Autodesk Inventor part; units mm, degrees
ref_plane "PulleyMidPlane1" through (-30.1251, 9, -4) normal (1, 0, 0) x (0, 0, -1)
ref_plane "PulleyMidPlane2" through (-23.3752, 9, -4) normal (1, 0, 0) x (0, 0, -1)
ref_plane "YZ Plane" through (0, 0, 0) normal (1, 0, 0) x (0, 1, 0)
sketch "Sketch1" plane through (0, 0, 0) normal (0, 1, 0) x (-1, 0, 0)
  line L0 (0, 0) -> (35.5, 0)
  line L1 (35.5, 0) -> (35.5, -90)
  line L2 (35.5, -90) -> (0, -90)
  line L3 (0, -90) -> (0, 0)
  dimension "d0" = 35.5
  dimension "d1" = 90
extrude "BlockShape" add sketch "Sketch1" along normal blind 9
sketch "Sketch3" plane through (0, 0, 0) normal (0, -1, 0) x (1, 0, 0)
  circle A0 centre (-10, -25) radius 3.25 construction
  line L0 (0, 0) -> (-35.5, 0)
  line L1 (-35.5, 0) -> (-35.5, -90)
  line L2 (-11.6286, -27.8125) -> (-13.25, -24.9958)
  line L3 (-13.25, -24.9958) -> (-11.6214, -22.1833)
  line L4 (-11.6214, -22.1833) -> (-8.3714, -22.1875)
  line L5 (-8.3714, -22.1875) -> (-6.75, -25.0042)
  line L6 (-6.75, -25.0042) -> (-8.3786, -27.8167)
  line L7 (-8.3786, -27.8167) -> (-11.6286, -27.8125)
  line L8 (0, -90) -> (0, 0)
  dimension "d15" = 6.5
  dimension "d16" = 25
  dimension "d26" = 10
extrude "SlideMountingNutWell1" cut sketch "Sketch3" against normal blind 5
sketch "Sketch5" plane through (0, 9, 0) normal (0, 1, 0) x (1, 0, 0)
  line L0 (0, 0) -> (0, 90)
  line L1 (-35.5, 0) -> (0, 0)
  circle A0 centre (-10, 25) radius 1.7
  circle A1 centre (-10, 15) radius 1.7
  dimension "d36" = 3.4
  dimension "d37" = 25
  dimension "d137" = 3.4
  dimension "d138" = 15
extrude "SlideMountingHoles" cut sketch "Sketch5" against normal through all
sketch "Sketch6" plane through (0, 9, 0) normal (0, 1, 0) x (1, 0, 0)
  line L0 (-32.5, 4) -> (-27.7502, 4)
  line L1 (-27.7502, 4) -> (-27.7502, 29.4)
  line L2 (-27.7502, 29.4) -> (-32.5, 29.4)
  line L3 (-32.5, 29.4) -> (-32.5, 4)
  line L4 (-35.5, 0) -> (0, 0)
  line L5 (-35.5, 90) -> (-35.5, 0)
  line L6 (-25.7502, 4) -> (-21.0002, 4)
  line L7 (-21.0002, 4) -> (-21.0002, 16.7)
  line L8 (-21.0002, 16.7) -> (-25.7502, 16.7)
  line L9 (-25.7502, 16.7) -> (-25.7502, 4)
  line L10 (0, 0) -> (0, 90) construction
  line L11 (-35.5, 90) -> (0, 90)
  line L12 (0, 0) -> (-20, 0) construction
  line L13 (-20, 0) -> (-20, 90) construction
  line L14 (-20, 90) -> (0, 90) construction
  line L15 (0, 90) -> (0, 0)
  circle A0 centre (-23.3752, 41.7) radius 1.7
  circle A1 centre (-30.125, 41.7) radius 1.7
  circle A2 centre (-30.125, 49.7) radius 1.7
  circle A3 centre (-23.3752, 49.7) radius 1.7
  dimension "d43" = 4.7498
  dimension "d44" = 25.4
  dimension "d45" = 4
  dimension "d46" = 3
  dimension "d47" = 4.75
  dimension "d48" = 2
  dimension "d49" = 20
  dimension "d50" = 3.4
  dimension "d90" = 3.4
  dimension "d91" = 5.375
  dimension "d92" = 3.4
  dimension "d93" = 8
  dimension "d94" = 3.4
  dimension "d99" = 40.3
extrude "Shape" cut sketch "Sketch6" against normal through all contours L3 L2 L1 L0 | L9 L8 L7 L6 | A0 | A1 | A2 | A3
sketch "Sketch7" plane through (0, 0, 0) normal (0, -1, 0) x (1, 0, 0)
  circle A0 centre (-23.3752, -41.7) radius 1.7
  circle A1 centre (-23.3752, -41.7) radius 3.25 construction
  line L0 (-23.3752, -38.45) -> (-20.5606, -40.075)
  line L1 (-20.5606, -40.075) -> (-20.5606, -43.325)
  line L2 (-20.5606, -43.325) -> (-23.3752, -44.95)
  line L3 (-23.3752, -44.95) -> (-26.1898, -43.325)
  line L4 (-26.1898, -43.325) -> (-26.1898, -40.075)
  line L5 (-26.1898, -40.075) -> (-23.3752, -38.45)
  line L6 (0, 0) -> (-35.5, 0)
  circle A2 centre (-30.125, -41.7) radius 3.25 construction
  line L7 (-35.5, 0) -> (-35.5, -90)
  line L8 (-30.1645, -44.9498) -> (-32.9591, -43.2907)
  line L9 (-32.9591, -43.2907) -> (-32.9196, -40.0409)
  line L10 (-32.9196, -40.0409) -> (-30.0855, -38.4502)
  line L11 (-30.0855, -38.4502) -> (-27.2909, -40.1093)
  line L12 (-27.2909, -40.1093) -> (-27.3304, -43.3591)
  line L13 (-27.3304, -43.3591) -> (-30.1645, -44.9498)
  dimension "d88" = 6.5
  dimension "d54" = 6.5
  dimension "d87" = 41.7
  dimension "d89" = 5.375
extrude "TensionNutWells1" cut sketch "Sketch7" against normal blind 5
sketch "Sketch8" plane through (-35.5, 0, -90) normal (-1, 0, 0) x (0, 0, 1)
  circle A0 centre (79.65, 4.5) radius 1.4605
  line L0 (0, 9) -> (90, 9)
  line L1 (90, 0) -> (90, 9)
  circle A1 centre (66.95, 4.5) radius 1.4605
  dimension "d57" = 2.921
  dimension "d58" = 4.5
  dimension "d59" = 10.35
  dimension "d103" = 2.921
  dimension "d104" = 4.5
  dimension "d105" = 12.7
hole "PulleyMountingHoles" at (-35.5, 4.5, -10.35) at (-35.5, 4.5, -23.05) direction (1, 0, 0) diameter 2.921 depth 22.5 counterbore diameter 3.4 counterbore depth 1.5
sketch "Sketch9" plane through (-21.0002, 9, -16.7) normal (-1, 0, 0) x (0, 0, 1)
  circle A0 centre (6.35, -4.5) radius 1.4605
  circle A1 centre (6.35, -4.5) radius 2.54
  point P0 (16.7, -9)
  dimension "d67" = 5.08
extrude "PulleyStandoff1" add sketch "Sketch9" along normal blind 0.2032
sketch "Sketch10" plane through (-27.7502, 9, -29.4) normal (-1, 0, 0) x (0, 0, 1)
  circle A0 centre (6.35, -4.5) radius 1.7
  circle A1 centre (6.35, -4.5) radius 2.54
  circle A2 centre (19.05, -4.5) radius 2.54
  circle A3 centre (19.05, -4.5) radius 2.54
  circle A4 centre (19.05, -4.5) radius 1.7
  point P0 (29.4, -9)
  dimension "d70" = 5.08
  dimension "d106" = 3.4
extrude "PulleyStandoff3" add sketch "Sketch10" along normal blind 0.2032
sketch "Sketch11" plane through (-25.7502, 9, -4) normal (1, 0, 0) x (0, 0, -1)
  circle A0 centre (6.35, -4.5) radius 1.7
  circle A1 centre (6.35, -4.5) radius 2.54
  point P0 (-4, -9)
  dimension "d73" = 5.08
extrude "PulleyStandoff2" add sketch "Sketch11" along normal blind 0.2032
sketch "Sketch12" plane through (-32.5, 9, -4) normal (1, 0, 0) x (0, 0, -1)
  circle A0 centre (6.35, -4.5) radius 1.7
  circle A1 centre (6.35, -4.5) radius 2.54
  circle A2 centre (19.05, -4.5) radius 1.4605
  circle A3 centre (19.05, -4.5) radius 2.54
  circle A4 centre (19.05, -4.5) radius 1.7
  point P0 (-4, -9)
  dimension "d76" = 5.08
  dimension "d107" = 5.08
  dimension "d108" = 3.4
extrude "PulleyStandof4" add sketch "Sketch12" along normal blind 0.2032 contours A1 | A3
sketch "Sketch14" plane through (0, 0, -90) normal (0, 0, -1) x (-1, 0, 0)
  circle A0 centre (18, 4.5) radius 2.25
  line L0 (35.5, 0) -> (0, 0)
  line L1 (0, 0) -> (0, 9)
  dimension "d82" = 4.5
  dimension "d83" = 4.5
  dimension "d84" = 18
extrude "4mmShaft" cut sketch "Sketch14" against normal blind 41
sketch "Sketch15" plane through (0, 9, 0) normal (0, 1, 0) x (1, 0, 0)
  circle A0 centre (-30.125, 49.7) radius 1.7
  circle A1 centre (-30.125, 49.7) radius 3.25 construction
  circle A2 centre (-23.3752, 49.7) radius 1.7
  circle A3 centre (-23.3752, 49.7) radius 3.25 construction
  line L0 (-30.125, 52.95) -> (-27.3104, 51.325)
  line L1 (-27.3104, 51.325) -> (-27.3104, 48.075)
  line L2 (-27.3104, 48.075) -> (-30.125, 46.45)
  line L3 (-30.125, 46.45) -> (-32.9396, 48.075)
  line L4 (-32.9396, 48.075) -> (-32.9396, 51.325)
  line L5 (-32.9396, 51.325) -> (-30.125, 52.95)
  line L6 (-23.3752, 52.95) -> (-20.5606, 51.325)
  line L7 (-20.5606, 51.325) -> (-20.5606, 48.075)
  line L8 (-20.5606, 48.075) -> (-23.3752, 46.45)
  line L9 (-23.3752, 46.45) -> (-26.1898, 48.075)
  line L10 (-26.1898, 48.075) -> (-26.1898, 51.325)
  line L11 (-26.1898, 51.325) -> (-23.3752, 52.95)
  point P0 (0, 0)
  dimension "d95" = 6.5
  dimension "d96" = 6.5
extrude "TensionNutWells2" cut sketch "Sketch15" against normal blind 5
ref_plane "PulleyMidPlane1" through (-30.1251, 9, -4) normal (1, 0, 0) x (0, 0, -1)
ref_plane "PulleyMidPlane2" through (-23.3752, 9, -4) normal (1, 0, 0) x (0, 0, -1)
sketch "Sketch20" plane through (0, 9, 0) normal (0, 1, 0) x (1, 0, 0)
  circle A0 centre (-29.5, 86) radius 1.524
  circle A1 centre (-29.5, 57.7) radius 1.524
  line L0 (-35.5, 90) -> (-35.5, 0)
  line L1 (0, 90) -> (-35.5, 90)
  circle A2 centre (-30.125, 49.7) radius 1.7
  point P0 (0, 0)
  dimension "d129" = 3.048
  dimension "d130" = 3.048
  dimension "d131" = 6
  dimension "d132" = 4
  dimension "d133" = 6
  dimension "d134" = 8
extrude "TieWrapHoles" cut sketch "Sketch20" against normal through all contours A0 | A1
sketch "Sketch21" plane through (0, 9, 0) normal (0, 1, 0) x (1, 0, 0)
  circle A0 centre (-10, 15) radius 1.7 construction
  circle A1 centre (-10, 15) radius 3.25 construction
  line L0 (-6.75, 15) -> (-8.375, 12.1854)
  line L1 (-8.375, 12.1854) -> (-11.625, 12.1854)
  line L2 (-11.625, 12.1854) -> (-13.25, 15)
  line L3 (-13.25, 15) -> (-11.625, 17.8146)
  line L4 (-11.625, 17.8146) -> (-8.375, 17.8146)
  line L5 (-8.375, 17.8146) -> (-6.75, 15)
  point P0 (0, 0)
  dimension "d139" = 6.5
extrude "SlideMountingNutWell2" cut sketch "Sketch21" against normal blind 5
sketch "Sketch22" plane through (0, 0, 0) normal (0, -1, 0) x (1, 0, 0)
  circle A0 centre (-9.525, -35) radius 1.9304 construction
  circle A1 centre (-9.525, -54.558) radius 1.9304 construction
  circle A2 centre (-10, -25) radius 1.7 construction
  line L0 (0, -90) -> (0, 0) construction
  dimension "d142" = 3.8608
  dimension "d143" = 3.8608
  dimension "d144" = 19.558
  dimension "d145" = 9.525
  dimension "d146" = 10
hole "XRrailMountingHoles1" at (-9.525, 0, -54.558) at (-9.525, 0, -35) direction (0, 1, 0) diameter 3.8608 end through all counterbore diameter 8.89 counterbore depth 3.048
sketch "Sketch23" plane through (0, 9, 0) normal (0, 1, 0) x (1, 0, 0)
  circle A0 centre (-9.525, 44.779) radius 1.9304 construction
  circle A1 centre (-9.525, 64.337) radius 1.9304 construction
  circle A2 centre (-9.525, 35) radius 1.9304
  line L0 (0, 0) -> (0, 90)
  dimension "d154" = 3.8608
  dimension "d155" = 3.8608
  dimension "d156" = 19.558
  dimension "d157" = 9.779
  dimension "d158" = 9.525
hole "XRrailMountingHoles2" at (-9.525, 9, -44.779) at (-9.525, 9, -64.337) direction (0, -1, 0) diameter 3.8608 end through all counterbore diameter 8.89 counterbore depth 3.048
sketch "Sketch25" plane through (0, 0, 0) normal (1, 0, 0) x (0, 0, -1)
  circle A0 centre (6.65, 4.5) radius 1.45
  line L0 (90, 0) -> (0, 0) construction
  line L1 (0, 9) -> (90, 9) construction
  line L2 (13.3, 4) -> (13.3, 0) construction
  line L3 (0, 0) -> (0, 9) construction
  line L4 (66.2674, 5.952) -> (62.4066, 5.952) construction
  line L5 (59.892, 9) -> (68.782, 9) construction
  line L6 (68.782, 5.952) -> (59.892, 5.952) construction
  line L7 (90, 0) -> (90, 9) construction
  circle A1 centre (75.8547, 4.5) radius 1.45
  circle A2 centre (82.9273, 4.5) radius 1.45
  dimension "d178" = 2.9
  dimension "d179" = 9
  dimension "d180" = 4.5
  dimension "d181" = 13.3
  dimension "d182" = 6.65
  dimension "d183" = 21.218
  dimension "d184" = 2.9
  dimension "d185" = 2.9
  dimension "d186" = 4.5
  dimension "d187" = 4.5
  dimension "d188" = 7.0727
  dimension "d189" = 7.0727
extrude "NonPulleySideHoles" cut sketch "Sketch25" against normal blind 13
sketch "Sketch26" plane through (-35.5, 0, -90) normal (-1, 0, 0) x (0, 0, 1)
  line L0 (60.6, 9) -> (60.6, 0) construction
  line L1 (51.5498, 0) -> (51.5498, 5) construction
  line L2 (33.824, 0) -> (30.776, 0) construction
  line L3 (5.524, 0) -> (2.476, 0) construction
  circle A0 centre (56.0749, 4.5) radius 1.45
  circle A1 centre (24.463, 4.5) radius 1.45
  line L4 (30.776, 9) -> (30.776, 0) construction
  line L5 (5.524, 9) -> (5.524, 0) construction
  line L6 (0, 9) -> (90, 9)
  circle A2 centre (18.15, 4.5) radius 1.45
  circle A3 centre (11.837, 4.5) radius 1.45
  point P0 (90, 0)
  dimension "d192" = 2.9
  dimension "d193" = 2.9
  dimension "d196" = 25.252
  dimension "d197" = 6.313
  dimension "d198" = 4.5
  dimension "d199" = 4.5
  dimension "d202" = 6.313
  dimension "d207" = 9.0502
  dimension "d208" = 4.5251
extrude "Extrusion17" cut sketch "Sketch26" against normal blind 13
equation "\"d133\" = d131"
equation "\"d157\" = 0.5 * d156"
equation "\"d158\" = d145"
equation "\"d180\" = 0.5 * d179"
equation "\"d182\" = 0.5 * d181"
equation "\"d186\" = d180"
equation "\"d187\" = d180"
equation "\"d188\" = 0.333333 * d183"
equation "\"d189\" = d188"
equation "\"d197\" = 0.25 * d196"
equation "\"d198\" = d180"
equation "\"d199\" = d180"
equation "\"d202\" = d197"
equation "\"d208\" = 0.5 * d207"
properties part number "Front fixed top coupler"
Could you check a few things on this model? Use its own coordinates, in mm. A direction names the side the tool comes from. Round coordinates to 2 decimals unless told otherwise and drop trailing zeros. Write each loop counter-clockwise with the first axis right and the second up, starting at its lowest first coordinate (ties: lowest second). Pieces come first, ordered by that corner, then holes. Notation, with made-up numbers: M -0.75,79 L 4.25,79 A25 ccw 4.25,107 Z; hole C -3.5,27 d7. An arc over 180 degrees is marked long. Answer in a Markdown table with one row per item. Add a question column.
Q1. On a 3-axis mill with a long thin cutter (end or side, diameter ignored), from which of +Z, -Z, +X, -X, +Y, -Y can I reach the whole of each face in a straight line? I mean faces 1 (the cylindrical face through (-6.41, 4.94, -8.03)), 2 (the flat face through (-29, 4, -48)), 3 (the cylindrical face through (-21.805, 7.028, -41.049)), 4 (the flat face through (-13, 4, -23)), 5 (the flat face through (-24.802, 2.465, -39.274)). Say none if no direction works.
Q2. If we mould it in two halves opening along Z, with no side actions, what happens to faces 6 (the flat face through (-18, 7, -90)), 7 (the flat face through (-7.57, 2.46, -23.58)), 8 (the cylindrical face through (-29.7, 4.56, -87.51))? For each: +Z half, -Z half, draft (parallel to the pull), parting line (faces both ways), or undercut.
Q3. Imagine slicing it at B-B (z = -34). Please give me the cut outline in (x, y), then the cut area to 3 significant figures.
Q4. Will these pins go through, and if not, where does the flat tip stop? pin 1 Ø11.5 at (x, z) = (-9.525, -44.779) entering from +Y; pin 2 Ø3 at (x, z) = (-24, -49) entering from +Y; pin 3 Ø1.5 at (y, z) = (5, -10) entering from -X; pin 4 Ø4.5 at (x, z) = (-30.125, -41.7) entering from -Y.
Q5. Imagine slicing it at C-C (z = -6). Please give me the cut outline in (x, y), then the cut area to 3 significant figures.
Q6. Imagine slicing it at A-A (x = -18). Please give me the cut outline in (y, z), then the cut area to 3 significant figures.
Q7. If I drill on line 1 (X direction, y = 2.5, z = -15); line 2 (X direction, y = 0.75, z = -11); line 3 (Z direction, x = -18.5, y = 4.5), over which ranges is the centre line in solid material (lowest first)? Write a range as from..to.
Values:
| question | item | result |
|---|---|---|
| 1 | face 1 | +X |
| 1 | face 2 | +Y |
| 1 | face 3 | +Y, -Y |
| 1 | face 4 | -X |
| 1 | face 5 | -Y |
| 2 | face 6 | -Z half |
| 2 | face 7 | undercut |
| 2 | face 8 | undercut |
| 3 | outline | M -35.5,0 L -13.86,0 L -13.86,3.05 L -11.18,3.05 L -11.18,9 L -35.5,9 L -35.5,5.95 L -22.5,5.95 L -22.5,3.05 L -35.5,3.05 Z; M -7.87,3.05 L -5.19,3.05 L -5.19,0 L 0,0 L 0,9 L -7.87,9 Z |
| 3 | area | 236 mm^2 |
| 4 | pin 1 | y = 9 |
| 4 | pin 2 | y = 4 |
| 4 | pin 3 | x = -13 |
| 4 | pin 4 | y = 5 |
| 5 | outline | M -35.5,0 L -32.5,0 L -32.5,9 L -35.5,9 Z; M -27.75,0 L -25.75,0 L -25.75,9 L -27.75,9 Z; M -21,0 L 0,0 L 0,3.2 L -13,3.2 L -13,5.8 L 0,5.8 L 0,9 L -21,9 Z |
| 5 | area | 200 mm^2 |
| 6 | outline | M 0,-90 L 2.25,-90 L 2.25,-49 L 6.75,-49 L 6.75,-90 L 9,-90 L 9,0 L 0,0 Z; hole C 4.5,-23.05 d2.92; hole C 4.5,-10.35 d2.92 |
| 6 | area | 612 mm^2 |
| 7 | line 1 | -35.5..-32.5, -27.75..-25.75, -21..-11.7, -8.3..0 |
| 7 | line 2 | -35.5..-32.5, -27.75..-25.75, -21..0 |
| 7 | line 3 | -49..-24.51, -21.59..-11.81, -8.89..0 |
